```python
from build123d import *

# Parameters (mm, degrees)
SKETCH105_W     = 48
SKETCH105_H     = 48
SKETCH105_R     = 1.7
PAD082_DEPTH    = 5
SKETCH106_W     = 10
SKETCH106_H     = 50
POCKET012_DEPTH = 3
SKETCH107_W     = 23.4
SKETCH107_H     = 23.4
POCKET013_DEPTH = 1.6
FILLET012_R     = 5
CHAMFER_ANGLE   = 45
CHAMFER_SIZE    = 1.3


with BuildPart() as part:
    # Sketch105 → Pad082 (new body)
    with BuildSketch(Plane.YZ):
        Rectangle(SKETCH105_W, SKETCH105_H)
        with Locations((19, 19)):
            Circle(SKETCH105_R, mode=Mode.SUBTRACT)
        with Locations((19, -19)):
            Circle(SKETCH105_R, mode=Mode.SUBTRACT)
        with Locations((-19, 19)):
            Circle(SKETCH105_R, mode=Mode.SUBTRACT)
        with Locations((-19, -19)):
            Circle(SKETCH105_R, mode=Mode.SUBTRACT)
    extrude(amount=PAD082_DEPTH)

    # Sketch106 (on DatumPlane) → Pocket012 (cut)
    with BuildSketch(Plane.YZ.offset(5)):
        with Locations((0, 15)):
            Rectangle(SKETCH106_W, SKETCH106_H)
    extrude(amount=-POCKET012_DEPTH, mode=Mode.SUBTRACT)

    # Sketch107 (on DatumPlane) → Pocket013 (cut)
    with BuildSketch(Plane.YZ.offset(5)):
        Rectangle(SKETCH107_W, SKETCH107_H)
    extrude(amount=-POCKET013_DEPTH, mode=Mode.SUBTRACT)

    # Fillet012
    fillet012_edges = [part.edges().sort_by_distance(p)[0] for p in [
        (2.5, 24, 24),
        (2.5, -24, 24),
        (2.5, -24, -24),
        (2.5, 24, -24),
    ]]
    fillet(fillet012_edges, radius=FILLET012_R)

    # Chamfer
    chamfer_edges = [part.edges().sort_by_distance(p)[0] for p in [
        (0, 17.3, 19),
        (0, -20.7, 19),
        (0, 17.3, -19),
        (0, -20.7, -19),
    ]]
    chamfer_side = part.faces().sort_by_distance((0, 0, 0))[0]
    chamfer(chamfer_edges, length=CHAMFER_SIZE, angle=CHAMFER_ANGLE, reference=chamfer_side)


solid = part.part
```
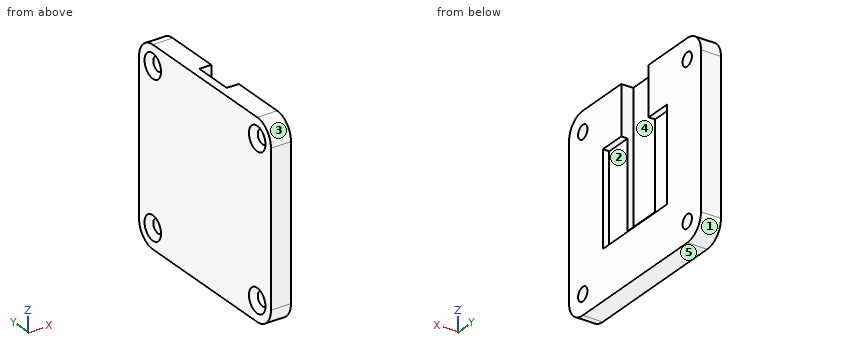
Design review of the part built by this model. Coordinates are the model's own, in mm. Face numbers are marked on the shaded views. A direction names the side the tool comes from. Coordinates: 2 decimals unless noted, no trailing zeros. Write each loop counter-clockwise with the first axis right and the second up, starting at its lowest first coordinate (ties: lowest second). Pieces come first, ordered by that corner, then holes.
1) To check wall thickness, follow L1, parallel to Z at x = 4.3, y = -19; L2, parallel to Z at x = 4.8, y = -9; L3, parallel to Y at x = 2.55, z = 13. State the ranges of each line that lie inside material, in increasing order.
2) Machinability: for the marked faces 1 and 2, which of the approach directions +Z, -Z, +X, -X, +Y, -Y give a long, thin tool a straight path to every point of the face, cutting with its end or side? Answer none if there is none.
3) Mouldability with a two-part tool opening along Y and no side actions: class the marked faces 3, 4 and 5 as +Y half, -Y half, draft (parallel to the pull), parting line (faces both ways), or undercut.
4) Add section A-A (z = 4). Write out the cut boundary in (x, y), plus the area to 3 significant figures.
5) Insertion check: pin 1 (1.5 mm diameter, centred on x = 3, y = 0.5, fed in from +Z); pin 2 (6 mm diameter, centred on y = -6.5, z = 11.5, fed in from +X); pin 3 (2.5 mm diameter, centred on y = -19, z = 19, fed in from +X); pin 4 (0.5 mm diameter, centred on x = 4.5, y = 3.5, fed in from +Z). Each pin has a flat end and moves straight along its axis. Give the tip position at first contact, or say it passes through.
Check result:
1. L1: z = -24 to -20.7, -17.3 to 17.3, 20.7 to 24
1. L2: z = -24 to -11.7, 11.7 to 24
1. L3: y = -24 to -5, 5 to 24
2. face 1: -Z, +X, -X, +Y
2. face 2: +X
3. face 3: -Y half
3. face 4: undercut
3. face 5: draft
4. outline: (0, -24) - (5, -24) - (5, -11.7) - (3.4, -11.7) - (3.4, -5) - (2, -5) - (2, 5) - (3.4, 5) - (3.4, 11.7) - (5, 11.7) - (5, 24) - (0, 24) - close
4. area: 189 mm2
5. pin 1: stops at z = -10
5. pin 2: stops at x = 5
5. pin 3: passes through
5. pin 4: stops at z = -11.7
